Part print with two shaded views. Sizes in mm from the minimum x, y, z corner. A direction names the side the tool comes from. Round coordinates to 2 decimals unless told otherwise and drop trailing zeros. Write each loop counter-clockwise with the first axis right and the second up, starting at its lowest first coordinate (ties: lowest second). Pieces come first, ordered by that corner, then holes. Notation, with made-up numbers: (76, 8) - (90, 8) arc R23 ccw to (90, 39) - close; hole circle Ø7 at (65.5, 68.25). An arc over 180 degrees is marked (long way). Answer as a JSON object with one key per item and string values. Group by question number.
Item 1: Slice it at D-D, the plane y = 3.75. List the corners of the cut face in (x, z).
Item 2: Slice it at B-B, the plane z = 22. List the corners of the cut face in (x, y).
Item 3: Two-plate mould, pull along Z, no slides. Class the marked faces 1, 2 and 3: +Z half, -Z half, draft (parallel to the pull), parting line (faces both ways), or undercut.
Item 4: Which spindle directions (+Z, -Z, +X, -X, +Y, -Y) get a long thin tool onto all of the face, cutting with end or side? Do the marked faces 4, 5 and 6. Say none if no direction does.
Item 5: Slice it at C-C, the plane y = 16.25. List the corners of the cut face in (x, z), then the cut area to 3 significant figures.
Item 6: Probe line 1 (Y direction, x = 22, z = 10); line 2 (X direction, y = 16.25, z = 22); line 3 (Y direction, x = 22.5, z = 13.5). List the from-to ranges inside material, lowest first. Write a range as from..to.
Item 7: Flat gauge pins, fed straight in: pin 1 (5 mm diameter, centred on x = 39.5, y = 23, fed in from -Z); pin 2 (8 mm diameter, centred on y = 15.5, z = 13, fed in from -X); pin 3 (6 mm diameter, centred on x = 14, y = 5, fed in from +Z). Where does each tip first touch, or does it go through?
Item 8: Slice it at A-A, the plane x = 22. List the corners of the cut face in (y, z), then the cut area to 3 significant figures.
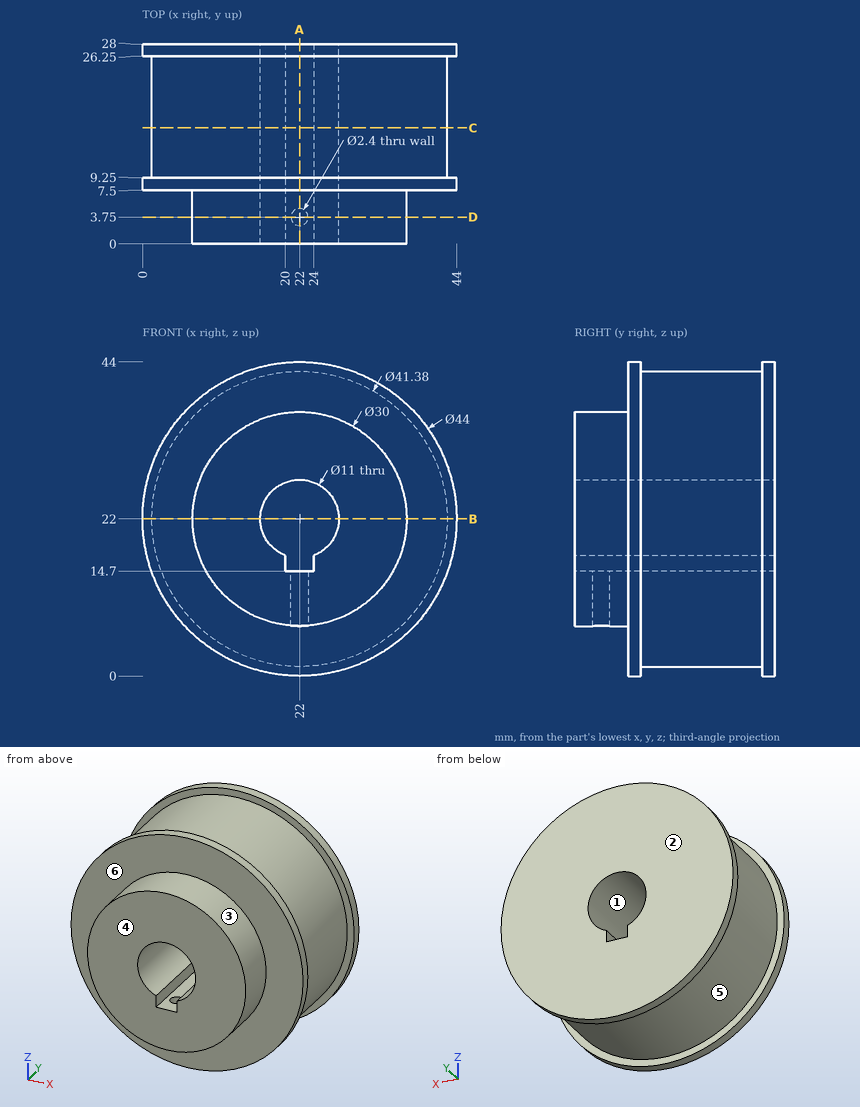
Geometry says:
{
 "1": {"outline": "(20, 14.7) - (20, 16.88) arc R5.5 cw (long way) to (24, 16.88) - (24, 14.7) - (23.2, 14.7) - (23.2, 7.05) arc R15 ccw (long way) to (20.8, 7.05) - (20.8, 14.7) - close"},
 "2": {"outline": "(0, 7.5) - (7, 7.5) - (7, 0) - (16.5, 0) - (16.5, 28) - (0, 28) - (0, 26.25) - (1.31, 26.25) - (1.31, 9.25) - (0, 9.25) - close; (27.5, 0) - (37, 0) - (37, 7.5) - (44, 7.5) - (44, 9.25) - (42.69, 9.25) - (42.69, 26.25) - (44, 26.25) - (44, 28) - (27.5, 28) - close"},
 "3": {"face 1": "undercut", "face 2": "draft", "face 3": "parting line"},
 "4": {"face 4": "+Z, -Z, +X, -X, -Y", "face 5": "none", "face 6": "-Y"},
 "5": {"outline": "circle Ø41.38 at (22, 22); hole (20, 14.7) - (24, 14.7) - (24, 16.88) arc R5.5 ccw (long way) to (20, 16.88) - close", "area": "1,240 mm^2"},
 "6": {"line 1": "y = 0..2.55, 4.95..28", "line 2": "x = 1.31..16.5, 27.5..42.69", "line 3": "y = 0..2.66, 4.84..28"},
 "7": {"pin 1": "stops at z = 7.75", "pin 2": "stops at x = 1.92", "pin 3": "stops at z = 43.07"},
 "8": {"outline": "(0, 7) - (2.55, 7) - (2.55, 14.7) - (0, 14.7) - close; (0, 27.5) - (28, 27.5) - (28, 44) - (26.25, 44) - (26.25, 42.69) - (9.25, 42.69) - (9.25, 44) - (7.5, 44) - (7.5, 37) - (0, 37) - close; (4.95, 7) - (7.5, 7) - (7.5, 0) - (9.25, 0) - (9.25, 1.31) - (26.25, 1.31) - (26.25, 0) - (28, 0) - (28, 14.7) - (4.95, 14.7) - close", "area": "706 mm^2"}
}
